Design review of the part built by this model. Coordinates are the model's own, in mm. Face numbers are marked on the shaded views. A direction names the side the tool comes from. Give positions to 0.01 mm unless a question says otherwise; leave off trailing zeros. Order: outer loops, then holes, each group sorted by start corner. A loop starts at its lowest first (then second) coordinate and runs counter-clockwise, first axis right, second up.
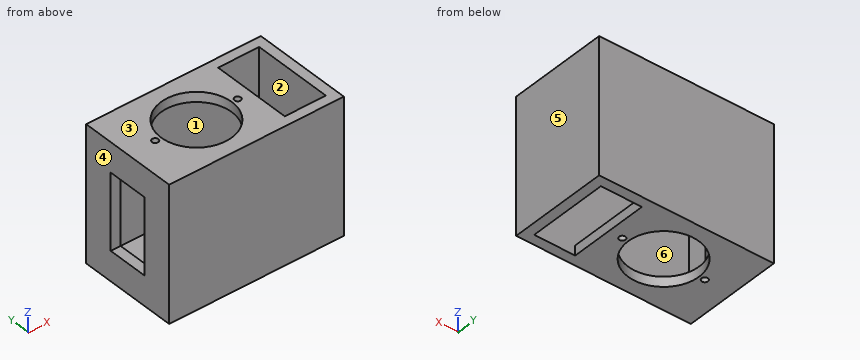
```python
from build123d import *

# Parameters (mm, degrees)
SKETCH1_W           = 88.9
SKETCH1_H           = 50.8
BOSS_EXTRUDE1_DEPTH = 68.58
SHELL5_START        = 5
SHELL5_OUTLINE_W    = 40.8
SHELL5_OUTLINE_H    = 58.58
SHELL5_DEPTH        = 78.9
SKETCH2_R           = 18
SKETCH2_R_2         = 1.6
SKETCH2_W           = 20.9
SKETCH2_H           = 40.8
CUT_EXTRUDE2_DEPTH  = 68.58
SKETCH7_W           = 38.58
SKETCH7_H           = 20.8
CUT_EXTRUDE6_DEPTH  = 10


# Read off the part's stored shape, not the designer's step: Shell5
with BuildPart() as part:
    # Sketch1 → Boss-Extrude1 (new body)
    with BuildSketch(Plane.XY):
        with Locations((44.45, 25.4)):
            Rectangle(SKETCH1_W, SKETCH1_H)
    extrude(amount=BOSS_EXTRUDE1_DEPTH)

    # Shell5 outline → Shell5 (cut)
    with BuildSketch(Plane.YZ.offset(SHELL5_START)):
        with Locations((25.4, 34.29)):
            Rectangle(SHELL5_OUTLINE_W, SHELL5_OUTLINE_H)
    extrude(amount=SHELL5_DEPTH, mode=Mode.SUBTRACT)

    # Sketch2 → Cut-Extrude2 (cut)
    with BuildSketch(Plane.XY.offset(68.58)):
        with Locations((35, 25.4)):
            Circle(SKETCH2_R)
        with Locations((14, 25.4)):
            Circle(SKETCH2_R_2)
        with Locations((56, 25.4)):
            Circle(SKETCH2_R_2)
        with Locations((73.45, 25.4)):
            Rectangle(SKETCH2_W, SKETCH2_H)
    extrude(amount=-CUT_EXTRUDE2_DEPTH, mode=Mode.SUBTRACT)

    # Sketch7 → Cut-Extrude6 (cut)
    with BuildSketch(Plane.ZY):
        with Locations((34.29, 25.4)):
            Rectangle(SKETCH7_W, SKETCH7_H)
    extrude(amount=-CUT_EXTRUDE6_DEPTH, mode=Mode.SUBTRACT)


solid = part.part
```
1. Take a section at A-A (x = 35). State the section outline as (y, z) points, then the cut area to 3 significant figures.
Recorded:
outline: (0, 0) - (7.4, 0) - (7.4, 5) - (5, 5) - (5, 63.58) - (7.4, 63.58) - (7.4, 68.58) - (0, 68.58) - close; (43.4, 0) - (50.8, 0) - (50.8, 68.58) - (43.4, 68.58) - (43.4, 63.58) - (45.8, 63.58) - (45.8, 5) - (43.4, 5) - close
area: 734 mm2
2. For pin 1 (1 mm diameter, centred on x = 47.5, z = 53, fed in from -Y), flat-tipped, find the tip position at first contact; note if it passes through.
Recorded:
pin 1: stops at y = 0
3. For line 1 along Y through (x, z) = (70, 45.5); line 2 along X through (y, z) = (9, 3.5); line 3 along Z through (x, y) = (55, 10), list the stretches that pass through material, from the lowest coordinate up.
Recorded:
line 1: y = 0 to 5, 45.8 to 50.8
line 2: x = 0 to 27.58, 42.42 to 63, 83.9 to 88.9
line 3: z = 0 to 5, 63.58 to 68.58
4. Take a section at C-C (y = 30.5). State the section outline as (x, z) points, then the cut area to 3 significant figures.
Recorded:
outline: (0, 0) - (17.74, 0) - (17.74, 5) - (5, 5) - (5, 15) - (0, 15) - close; (0, 53.58) - (5, 53.58) - (5, 63.58) - (17.74, 63.58) - (17.74, 68.58) - (0, 68.58) - close; (52.26, 0) - (63, 0) - (63, 5) - (52.26, 5) - close; (52.26, 63.58) - (63, 63.58) - (63, 68.58) - (52.26, 68.58) - close; (83.9, 0) - (88.9, 0) - (88.9, 68.58) - (83.9, 68.58) - close
area: 728 mm2
5. Machinability: for the marked faces 1, 2 and 3, which of the approach directions +Z, -Z, +X, -X, +Y, -Y give a long, thin tool a straight path to every point of the face, cutting with its end or side? Answer none if there is none.
Recorded:
face 1: none
face 2: +Z, -Z
face 3: +Z, +X, -X, +Y, -Y
6. Take a section at D-D (y = 40). State the section outline as (x, z) points.
Recorded:
outline: (0, 0) - (24.47, 0) - (24.47, 5) - (5, 5) - (5, 63.58) - (24.47, 63.58) - (24.47, 68.58) - (0, 68.58) - close; (45.53, 0) - (63, 0) - (63, 5) - (45.53, 5) - close; (45.53, 63.58) - (63, 63.58) - (63, 68.58) - (45.53, 68.58) - close; (83.9, 0) - (88.9, 0) - (88.9, 68.58) - (83.9, 68.58) - close
7. Take a section at B-B (z = 62.5). State the section outline as (x, y) points.
Recorded:
outline: (0, 0) - (88.9, 0) - (88.9, 50.8) - (0, 50.8) - close; hole (5, 5) - (83.9, 5) - (83.9, 45.8) - (5, 45.8) - close
8. Draft analysis for pull direction X (two halves, no side actions). For the marked faces 4, 5 and 6, state which applies: pulls with the +X half, pulls with the -X half, needs draft (parallel to the pull), parting line crosses it, or undercut.
Recorded:
face 4: pulls with the -X half
face 5: pulls with the +X half
face 6: undercut
